Geometry check sheet. Reference: drawing and pictorial views, mm from the part's lowest x, y, z. Round coordinates to 2 decimals unless told otherwise and drop trailing zeros. Loops run counter-clockwise (first coordinate to the right, second up) from the corner with the lowest first, then second, coordinate; pieces in that order, holes last. Notation, with made-up numbers: (69, 8) - (75, 8) arc R20 ccw to (75, 14) - close; hole circle Ø10 at (27, 37.5). An arc over 180 degrees is marked (long way). Put each result on its own line as item: value. Start each with the question number.
Item 1: Gauge pin test, flat ends, axial feed: pin 1 Ø8 at (x, z) = (24, 4) entering from +Y (1 decimal); pin 2 Ø9.5 at (x, z) = (18.1, 11.35) entering from +Y; pin 3 Ø4 at (y, z) = (27, 9) entering from -X; pin 4 Ø10 at (x, z) = (26.5, 10) entering from +Y (1 decimal). Record the tip position at first contact, or that the pin passes through.
Item 2: Material ranges on line 1 along Z through (x, y) = (11.5, 18) (1 decimal); line 2 along Z through (x, y) = (16, 2.5) (1 decimal); line 3 along Y through (x, z) = (2, 10.5) (1 decimal), recorded low to high.
Item 3: Draft check along Y on the marked faces 1, 2, 3 and 4. Enter one of: pulls with the +Y half, pulls with the -Y half, needs draft (parallel to the pull), parting line crosses it, or undercut.
Item 4: Section check B-B, the plane z = 18.5. Record the cut outline in (x, y) (1 decimal), and give its area (3 significant figures).
Item 5: Section check A-A, the plane z = 14.25. Give the number of separate pieces and of enclosed holes in the cut face, and give its area (3 significant figures).
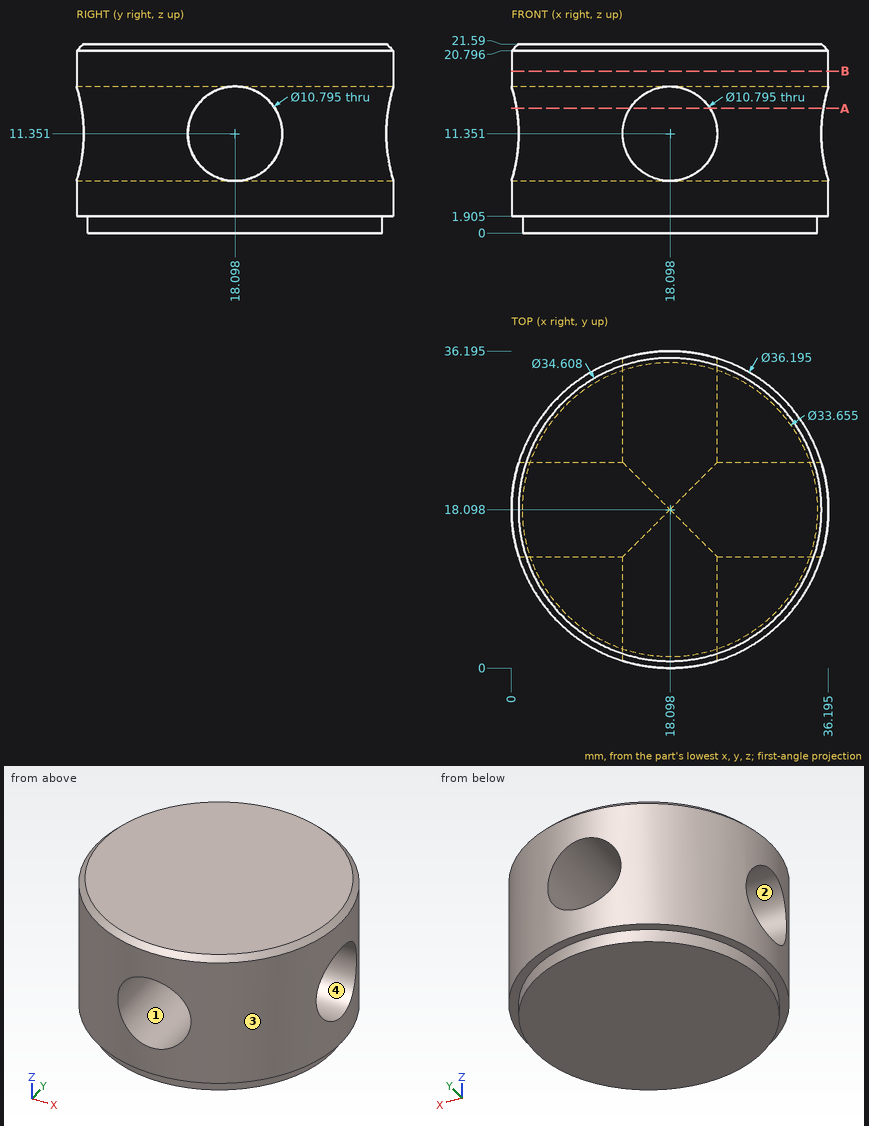
Check result:
1. pin 1: y = 36.1
1. pin 2: through
1. pin 3: x = 1.37
1. pin 4: y = 35.8
2. line 1: 0 to 6, 16.7 to 21.6
2. line 2: 0 to 6.4, 16.3 to 21.6
2. line 3: 9.8 to 12.8, 23.4 to 26.4
3. face 1: needs draft
3. face 2: undercut
3. face 3: parting line crosses it
3. face 4: undercut
4. outline: circle Ø36.2 at (18.1, 18.1)
4. area: 1,030 mm²
5. separate pieces: 4
5. enclosed holes: 0
5. area: 460 mm²
